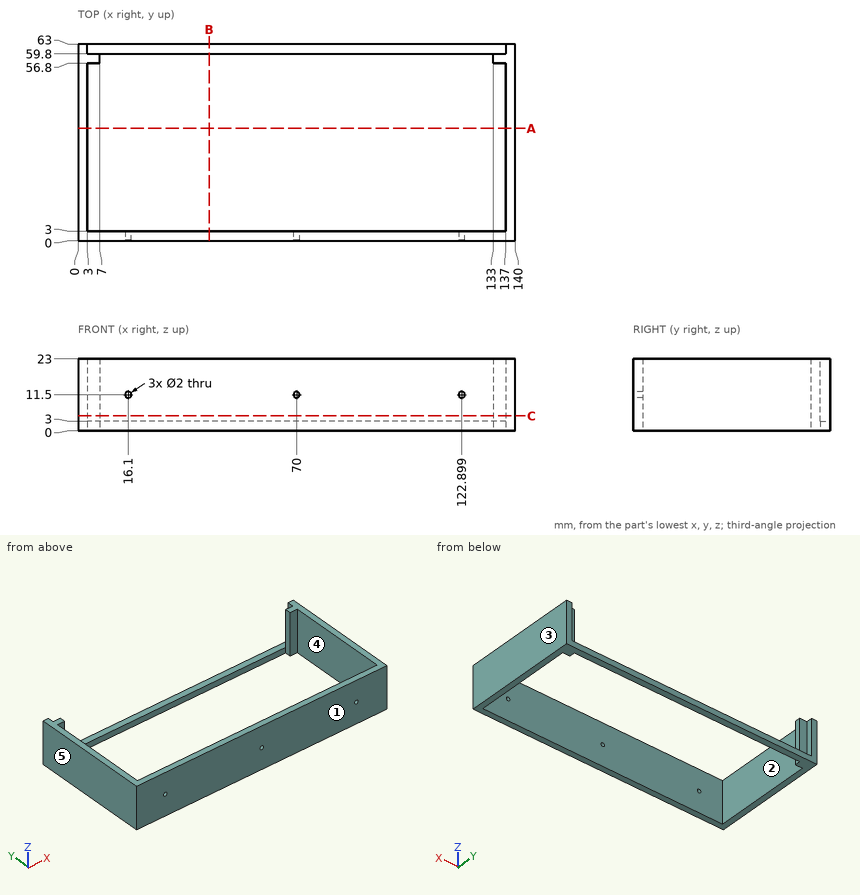
Here's the drawing with two shaded views (mm, measured from the low corner). I have some questions. A direction names the side the tool comes from. Give positions to 0.01 mm unless a question says otherwise; leave off trailing zeros. Order: outer loops, then holes, each group sorted by start corner. A loop starts at its lowest first (then second) coordinate and runs counter-clockwise, first axis right, second up. Notation, with made-up numbers: (-25.75, 3.5) -> (-1.75, 3.5) arc R12 ccw to (-1.75, 8.5) -> close; hole circle Ø1 at (14.25, 63). An arc over 180 degrees is marked (long way). One line per item, written item: value. Start each with the question number.
1. Imagine slicing it at A-A, the plane y = 36. List the corners of the cut face in (x, z) for me.
2. Imagine slicing it at B-B, the plane x = 42. List the corners of the cut face in (y, z) for me.
3. I need wall thicknesses on probe 1 along X at (y, z) = (6.5, 4); probe 2 along Z at (x, y) = (70, 1.45); probe 3 along X at (y, z) = (59.5, 3). Which ranges of each line are inside material? Lowest first, please. Write a range as from..to.
4. We'd pull the mould along X, two halves only. Please class the marked faces 3, 4 and 5: released by +X, released by -X, zero draft, split by the parting line, or undercut.
5. Imagine slicing it at C-C, the plane z = 4.75. List the corners of the cut face in (x, y) for me, plus the area to 3 significant figures.
6. Will these pins go through, and if not, where does the flat tip stop? pin 1 Ø4.5 at (x, z) = (134.5, 11.5) entering from +Y; pin 2 Ø1.2 at (x, z) = (70, 11.5) entering from +Y; pin 3 Ø1 at (x, y) = (80.5, 61) entering from +Z; pin 4 Ø2.5 at (y, z) = (61, 13.5) entering from -X.
7. For the marked faces 1 and 2, which set-ups out of +Z, -Z, +X, -X, +Y, -Y let a thin tool reach every point of the face, with its end or its side?
Values follow:
1. outline: (0, 0) -> (3, 0) -> (3, 23) -> (0, 23) -> close; (137, 0) -> (140, 0) -> (140, 23) -> (137, 23) -> close
2. outline: (0, 0) -> (3, 0) -> (3, 23) -> (0, 23) -> close; (59.8, 0) -> (63, 0) -> (63, 3) -> (59.8, 3) -> close
3. probe 1: x = 0..3, 137..140
3. probe 2: z = 0..10.5, 12.5..23
3. probe 3: x = 0..7, 133..140
4. face 3: released by +X
4. face 4: undercut
4. face 5: released by -X
5. outline: (0, 0) -> (140, 0) -> (140, 63) -> (137, 63) -> (137, 59.8) -> (133, 59.8) -> (133, 56.8) -> (137, 56.8) -> (137, 3) -> (3, 3) -> (3, 56.8) -> (7, 56.8) -> (7, 59.8) -> (3, 59.8) -> (3, 63) -> (0, 63) -> close
5. area: 804 mm2
6. pin 1: stops at y = 59.8
6. pin 2: passes through
6. pin 3: stops at z = 3
6. pin 4: stops at x = 0
7. face 1: +Z, -Z, +X, -X, -Y
7. face 2: +Z, -Z
